Geometry check sheet. Reference: drawing and pictorial views, mm from the part's lowest x, y, z. Round coordinates to 2 decimals unless told otherwise and drop trailing zeros. Write each loop counter-clockwise with the first axis right and the second up, starting at its lowest first coordinate (ties: lowest second). Pieces come first, ordered by that corner, then holes. Notation, with made-up numbers: (19.5, 54.25) -> (65.5, 54.25) arc R31 cw to (65.5, 93.25) -> close; hole circle Ø1 at (49, 85.5). An arc over 180 degrees is marked (long way). Answer as a JSON object with one key per item and string values. Group by question number.
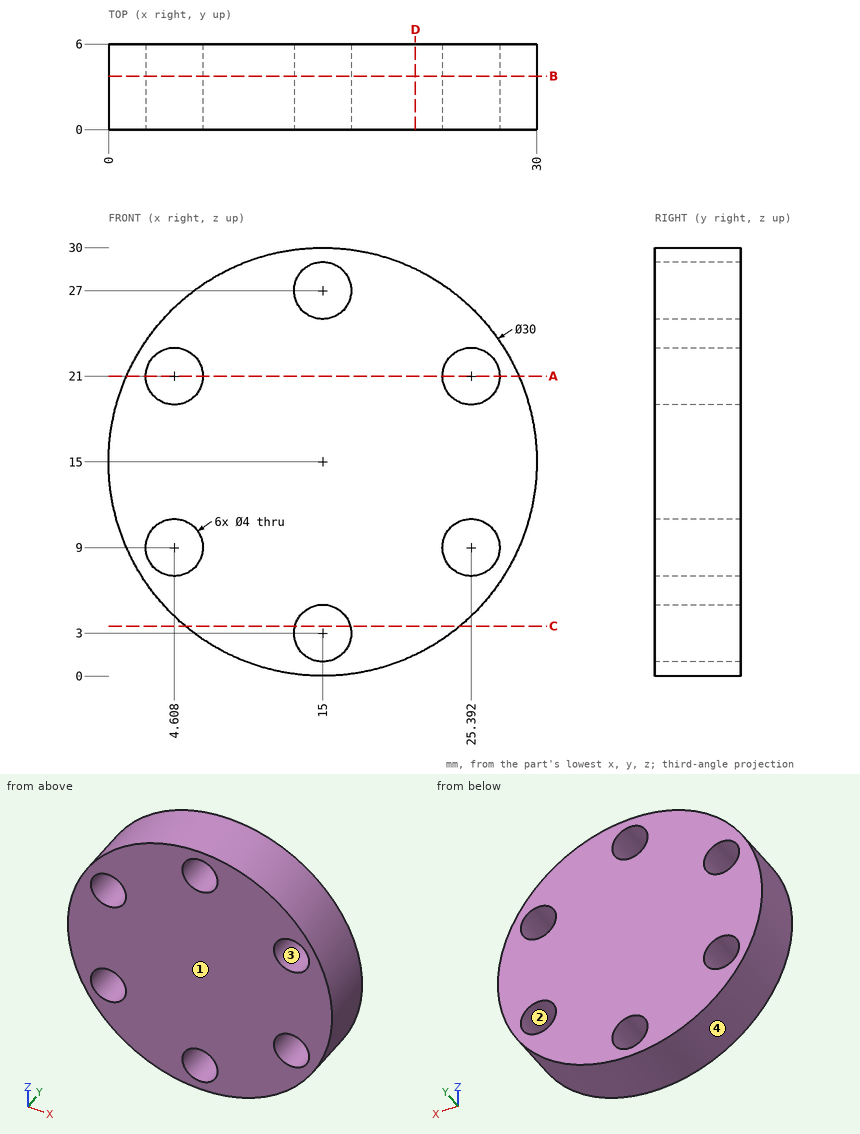
(1) Go/stop test with a flat-tipped pin: pin 1 Ø3 at (x, y) = (4, 0.5) entering from +Z. Record where the tip stops, or that it passes through.
(2) Release check for a two-part mould opening along Z. For the marked faces 1, 2, 3 and 4 record: pulls with the +Z half, pulls with the -Z half, needs draft (parallel to the pull), parting line crosses it, or undercut.
(3) Scan lines: line 1 along X through (y, z) = (4.5, 21); line 2 along Z through (x, y) = (27, 0.6); line 3 along Z through (x, y) = (15.5, 5.2). Record each from-to range of solid material in increasing order.
(4) Section check B-B on y = 3.75. Record the cut outline in (x, z).
(5) Section check D-D on x = 21.5. Record the cut outline in (y, z), then the cut area to 3 significant figures.
(6) Section check A-A on z = 21. Record the cut outline in (x, y).
(7) Section check C-C on z = 3.5. Record the cut outline in (x, y).
Data:
{
 "1": {"pin 1": "stops at z = 26.61"},
 "2": {"face 1": "needs draft", "face 2": "undercut", "face 3": "undercut", "face 4": "parting line crosses it"},
 "3": {"line 1": "x = 1.25 to 2.61, 6.61 to 23.39, 27.39 to 28.75", "line 2": "z = 6 to 7.81, 10.19 to 19.81, 22.19 to 24", "line 3": "z = 0.01 to 1.06, 4.94 to 25.06, 28.94 to 29.99"},
 "4": {"outline": "circle Ø30 at (15, 15); hole circle Ø4 at (4.61, 9); hole circle Ø4 at (4.61, 21); hole circle Ø4 at (15, 3); hole circle Ø4 at (15, 27); hole circle Ø4 at (25.39, 9); hole circle Ø4 at (25.39, 21)"},
 "5": {"outline": "(0, 1.48) -> (6, 1.48) -> (6, 28.52) -> (0, 28.52) -> close", "area": "162 mm²"},
 "6": {"outline": "(1.25, 0) -> (2.61, 0) -> (2.61, 6) -> (1.25, 6) -> close; (6.61, 0) -> (23.39, 0) -> (23.39, 6) -> (6.61, 6) -> close; (27.39, 0) -> (28.75, 0) -> (28.75, 6) -> (27.39, 6) -> close"},
 "7": {"outline": "(5.37, 0) -> (13.06, 0) -> (13.06, 6) -> (5.37, 6) -> close; (16.94, 0) -> (24.63, 0) -> (24.63, 6) -> (16.94, 6) -> close"}
}
